Source: CAD feature listing. Evaluate the final solid. Frame: model axes, mm. A direction names the side the tool comes from. Give positions to 0.01 mm unless a question says otherwise; leave off trailing zeros. Loops run counter-clockwise (first coordinate to the right, second up) from the corner with the lowest first, then second, coordinate; pieces in that order, holes last. Notation, with made-up numbers: M -29.5,-21 L -17.5,-21 A29 ccw -17.5,14 Z; hole C 21,37 d10. An arc over 180 degrees is marked long. Put each result on its own line as item: value. Start each with the question number.
```python
from build123d import *

# Parameters (mm, degrees)
ESBO_O1_W                = 10
ESBO_O1_H                = 25
RESSALTO_EXTRUS_O1_DEPTH = 8
ESBO_O2_W                = 6.7
ESBO_O2_H                = 14.3
CORTE_EXTRUS_O1_DEPTH    = 3
ESBO_O3_W                = 5
ESBO_O3_H                = 8
RESSALTO_EXTRUS_O2_DEPTH = 3
ESBO_O5_R                = 1.25
CORTE_EXTRUS_O2_DEPTH    = 26.455844123
FILETE1_R                = 3
FILETE1_OF_ESPELHAR3_R   = 3
ESBO_O6_W                = 5.1
ESBO_O6_H                = 12.7
CORTE_EXTRUS_O3_DEPTH    = 3
ESBO_O7_R                = 2
CORTE_EXTRUS_O4_DEPTH    = 18.095320997
FILETE2_R                = 3


with BuildPart() as part:
    # Esboço1 → Ressalto-extrusão1 (new body)
    with BuildSketch(Plane(origin=(0, 0, 0), x_dir=(1, 0, 0), z_dir=(0, 1, 0))):
        Rectangle(ESBO_O1_W, ESBO_O1_H)
    extrude(amount=RESSALTO_EXTRUS_O1_DEPTH)

    # Esboço2 → Corte-extrusão1 (cut)
    with BuildSketch(Plane(origin=(0, 8, 0), x_dir=(1, 0, 0), z_dir=(0, 1, 0))):
        with Locations((0, -3.85)):
            Rectangle(ESBO_O2_W, ESBO_O2_H)
    extrude(amount=-CORTE_EXTRUS_O1_DEPTH, mode=Mode.SUBTRACT)

    # Esboço3 → Ressalto-extrusão2 (add)
    with BuildSketch(Plane(origin=(0, 0, -12.5), x_dir=(-1, 0, 0), z_dir=(0, 0, -1))):
        with Locations((-7.5, 4)):
            Rectangle(ESBO_O3_W, ESBO_O3_H)
    ressalto_extrus_o2 = extrude(amount=-RESSALTO_EXTRUS_O2_DEPTH)

    # Esboço5 → Corte-extrusão2 (cut, through all)
    with BuildSketch(Plane.XY.offset(-9.5)):
        with Locations((7.5, 4)):
            Circle(ESBO_O5_R)
    corte_extrus_o2 = extrude(amount=-CORTE_EXTRUS_O2_DEPTH, mode=Mode.SUBTRACT)

    # Filete1
    filete1_edges = [part.edges().sort_by_distance(p)[0] for p in [
        (10, 0, -11),
        (10, 8, -11),
    ]]
    fillet(filete1_edges, radius=FILETE1_R)

    # Espelhar3: Ressalto-extrusão2, Corte-extrusão2 across plane
    add(ressalto_extrus_o2.mirror(Plane(origin=(0, 0, 0), x_dir=(0, 0, 1), z_dir=(1, 0, 0))))
    add(corte_extrus_o2.mirror(Plane(origin=(0, 0, 0), x_dir=(0, 0, 1), z_dir=(1, 0, 0))), mode=Mode.SUBTRACT)

    # Filete1 of Espelhar3
    filete1_of_espelhar3_edges = [part.edges().sort_by_distance(p)[0] for p in [
        (-10, 0, -11),
        (-10, 8, -11),
    ]]
    fillet(filete1_of_espelhar3_edges, radius=FILETE1_OF_ESPELHAR3_R)

    # Esboço6 → Corte-extrusão3 (cut)
    with BuildSketch(Plane(origin=(0, 5, 0), x_dir=(1, 0, 0), z_dir=(0, 1, 0))):
        with Locations((0, -3.85)):
            Rectangle(ESBO_O6_W, ESBO_O6_H)
    extrude(amount=-CORTE_EXTRUS_O3_DEPTH, mode=Mode.SUBTRACT)

    # Esboço7 → Corte-extrusão4 (cut, through all)
    with BuildSketch(Plane(origin=(0, 2, 0), x_dir=(1, 0, 0), z_dir=(0, 1, 0))):
        with Locations(Location((0, -0.5, 0), (0, 0, 270))):
            Circle(ESBO_O7_R)
    extrude(amount=-CORTE_EXTRUS_O4_DEPTH, mode=Mode.SUBTRACT)

    # Filete2
    filete2_edges = [part.edges().sort_by_distance(p)[0] for p in [
        (0, 0, 12.5),
        (5, 4, 12.5),
        (-5, 4, 12.5),
    ]]
    fillet(filete2_edges, radius=FILETE2_R)


solid = part.part
```
1. Section C-C, the plane z = -10.25. Output: boundary loops of the cut face in (x, y), plus the area to 3 significant figures.
2. Contact query for flat-ended pins moving along their axis: pin 1 (4 mm diameter, centred on y = 6, z = -0.5, fed in from -X); pin 2 (2.5 mm diameter, centred on y = 2.5, z = 3, fed in from +X); pin 3 (8 mm diameter, centred on x = 7.5, z = -3, fed in from +Y); pin 4 (4.5 mm diameter, centred on x = 0, z = 0.5, fed in from +Y). Output: stop coordinate, or through.
3. Set-up query: faces 4 (the face through (-1.774, 1.014, 1.423)), 5 (the face through (3, 5, 3)). Return all of +Z, -Z, +X, -X, +Y, -Y with unobstructed straight access to the full face (end or side cutting, diameter ignored); none if empty.
4. Pull-direction query (Z, two-part tool) for faces 1 (the face through (-10, 4, -11)), 2 (the face through (6, 3, -9.5)), 3 (the face through (0, 7, -3.3)); classes: released by +Z, released by -Z, zero draft, split by the parting line, or undercut.
5. Ray query, line 1 (X direction, y = 3.5, z = 2.25); line 2 (X direction, y = 6, z = 5); line 3 (X direction, y = 4, z = -7). Return the intervals inside material, ascending.
6. Section B-B, the plane y = 4. Output: boundary loops of the cut face in (x, z).
7. Section A-A, the plane z = 0.5. Output: boundary loops of the cut face in (x, y).
8. Section D-D, the plane x = 7.5. Output: boundary loops of the cut face in (y, z), plus the area to 3 significant figures.
Results found:
1. outline: M -10,3 A3 ccw -7,0 L 7,0 A3 ccw 10,3 L 10,5 A3 ccw 7,8 L -7,8 A3 ccw -10,5 Z; hole C -7.5,4 d2.5; hole C 7.5,4 d2.5
1. area: 142 mm²
2. pin 1: x = -5
2. pin 2: x = 5
2. pin 3: y = 8
2. pin 4: y = 2
3. face 4: +Y, -Y
3. face 5: +Y
4. face 1: zero draft
4. face 2: released by +Z
4. face 3: undercut
5. line 1: -5 to -2.55, 2.55 to 5
5. line 2: -5 to -3.35, 3.35 to 5
5. line 3: -5 to 5
6. outline: M -10,-12.5 L -8.75,-12.5 L -8.75,-9.5 L -10,-9.5 Z; M -6.25,-12.5 L 6.25,-12.5 L 6.25,-9.5 L 5,-9.5 L 5,9.5 A3 ccw 2,12.5 L -2,12.5 A3 ccw -5,9.5 L -5,-9.5 L -6.25,-9.5 Z; M 8.75,-12.5 L 10,-12.5 L 10,-9.5 L 8.75,-9.5 Z; hole M -2.55,-2.5 L 2.55,-2.5 L 2.55,10.2 L -2.55,10.2 Z
7. outline: M -5,0 L -2,0 L -2,2 L -2.55,2 L -2.55,5 L -3.35,5 L -3.35,8 L -5,8 Z; M 2,0 L 5,0 L 5,8 L 3.35,8 L 3.35,5 L 2.55,5 L 2.55,2 L 2,2 Z
8. outline: M 0.04,-12.5 L 2.75,-12.5 L 2.75,-9.5 L 0.04,-9.5 Z; M 5.25,-12.5 L 7.96,-12.5 L 7.96,-9.5 L 5.25,-9.5 Z
8. area: 16.2 mm²
